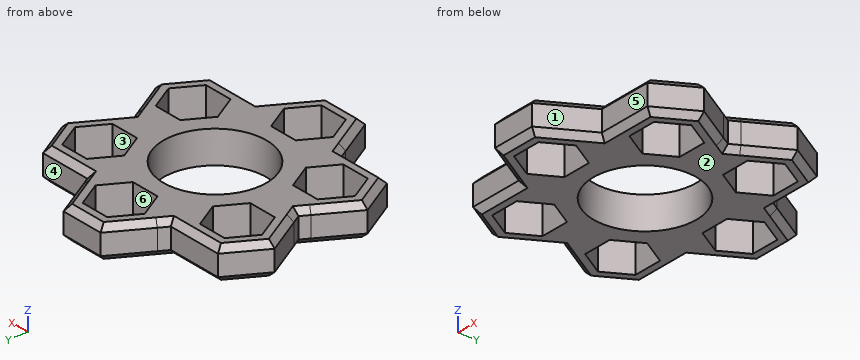
from build123d import *

# Parameters (mm, degrees)
F1_DEPTH = 6.9977
F2_R     = 11.176
F3_DEPTH = 6.9977
F4_SIZE  = 1.27


# Not quite as in the source:
# - a feature names something its author has since deleted; it is built from what else it names


with BuildPart() as f1:
    # F0 (on Top) → F1 (new body)
    with BuildSketch(Plane.XY):
        Polygon((-1.27, 12.7), (1.27, 12.7), (5.4871048633, 12.7), (6.9125849394, 15.169003917), (7.0907659214, 15.4776224307), (9.8865139145, 20.32), (5.1204874424, 28.575), (-4.411565502, 28.575), (-9.1775919741, 20.32), (-4.7781829229, 12.7), align=None)
        Polygon((6.6602806103, 20.32), (3.5073707902, 14.859), (-2.7984488498, 14.859), (-5.9513586699, 20.32), (-2.7984488498, 25.781), (3.5073707902, 25.781), align=None, mode=Mode.SUBTRACT)
        Polygon((6.9125849394, 15.169003917), (5.4871048633, 12.7), (7.3323484187, 12.7), (8.4322006815, 10.795), (12.8316097327, 18.415), (10.9863661773, 18.415), (9.8865139145, 20.32), (7.0907659214, 15.4776224307), align=None)
        Polygon((-7.3323484187, 12.7), (-4.7781829229, 12.7), (-9.1775919741, 20.32), (-10.3250266623, 18.3325848218), (-12.8789355329, 18.3325848218), (-8.4796547943, 10.7128070657), align=None)
        Polygon((12.8316097327, 18.415), (8.4322006815, 10.795), (11.6335226281, 5.2501477372), (13.5648445746, 1.905), (16.3276362049, 1.905), (18.8676362049, 1.905), (22.3636626771, 1.905), (27.1296891492, 10.16), (22.3636626771, 18.415), align=None)
        Polygon((20.7505460249, 4.699), (14.4447263849, 4.699), (11.2918165648, 10.16), (14.4447263849, 15.621), (20.7505460249, 15.621), (23.903455845, 10.16), align=None, mode=Mode.SUBTRACT)
        Polygon((-9.8614826635, 8.3194109889), (-8.4796547943, 10.7128070657), (-12.8789355329, 18.3325848218), (-22.4109884772, 18.3325848218), (-27.1770149494, 10.0775848218), (-22.4109884772, 1.8225848218), (-13.612427, 1.8225848218), (-11.1783483187, 6.0385327673), align=None)
        Polygon((-14.492052185, 15.5385848218), (-11.339142365, 10.0775848218), (-14.492052185, 4.6165848218), (-20.7978718251, 4.6165848218), (-23.9507816452, 10.0775848218), (-20.7978718251, 15.5385848218), align=None, mode=Mode.SUBTRACT)
        Polygon((16.3276362049, 1.905), (13.5648445746, 1.905), (14.6646968374, 0), (13.5648445746, -1.905), (22.3636626771, -1.905), (21.2638104143, 0), (22.3636626771, 1.905), (18.8676362049, 1.905), align=None)
        Polygon((-14.6646968374, 0), (-13.612427, 1.8225848218), (-22.4109884772, 1.8225848218), (-21.311264527, -0.0821929343), (-22.3636626771, -1.905), (-19.9342235854, -1.905), (-17.3764717744, -1.905), (-13.5648445746, -1.905), align=None)
        Polygon((22.3636626771, -1.905), (13.5648445746, -1.905), (10.3635226281, -7.4498522628), (8.4322006815, -10.795), (9.8135964967, -13.1876477372), (11.0835964967, -15.3873522628), (12.8316097327, -18.415), (22.3636626771, -18.415), (27.1296891492, -10.16), align=None)
        Polygon((14.4447263849, -15.621), (11.2918165648, -10.16), (14.4447263849, -4.699), (20.7505460249, -4.699), (23.903455845, -10.16), (20.7505460249, -15.621), align=None, mode=Mode.SUBTRACT)
        Polygon((-11.6335226281, -5.2501477372), (-13.5648445746, -1.905), (-17.3764717744, -1.905), (-19.9342235854, -1.905), (-22.3636626771, -1.905), (-27.1296891492, -10.16), (-22.3636626771, -18.415), (-12.8316097327, -18.415), (-8.4322006815, -10.795), (-10.3635226281, -7.4498522628), align=None)
        Polygon((-20.7505460249, -4.699), (-14.4447263849, -4.699), (-11.2918165648, -10.16), (-14.4447263849, -15.621), (-20.7505460249, -15.621), (-23.903455845, -10.16), align=None, mode=Mode.SUBTRACT)
        Polygon((9.8135964967, -13.1876477372), (8.4322006815, -10.795), (7.3323484187, -12.7), (5.1326438931, -12.7), (9.5320529443, -20.32), (4.7660264722, -28.575), (10.6457036946, -18.415), (12.8316097327, -18.415), (11.0835964967, -15.3873522628), align=None)
        Polygon((9.5320529443, -20.32), (5.1326438931, -12.7), (1.27, -12.7), (-1.27, -12.7), (-5.1326438931, -12.7), (-6.5140397082, -15.0926477372), (-7.7840397082, -17.2923522628), (-9.5320529443, -20.32), (-4.7660264722, -28.575), (4.7660264722, -28.575), align=None)
        Polygon((-6.3058196401, -20.32), (-3.15290982, -14.859), (3.15290982, -14.859), (6.3058196401, -20.32), (3.15290982, -25.781), (-3.15290982, -25.781), align=None, mode=Mode.SUBTRACT)
        Polygon((-7.3323484187, -12.7), (-8.4322006815, -10.795), (-12.8316097327, -18.415), (-10.6319052071, -18.415), (-9.5320529443, -20.32), (-7.7840397082, -17.2923522628), (-6.5140397082, -15.0926477372), (-5.1326438931, -12.7), align=None)
        Polygon((5.4871048633, 12.7), (1.27, 12.7), (-1.27, 12.7), (-4.7781829229, 12.7), (-4.411565502, 12.065), (-2.0086818804, 12.065), (1.267424375, 12.065), (5.1204874424, 12.065), align=None)
        Polygon((-12.8316097327, -1.905), (-13.5648445746, -1.905), (-11.6335226281, -5.2501477372), (-11.0835964967, -4.9326477372), align=None)
        Polygon((1.27, -12.7), (5.1326438931, -12.7), (4.7660264722, -12.065), (1.27, -12.065), (-1.27, -12.065), (-4.7660264722, -12.065), (-5.1326438931, -12.7), (-1.27, -12.7), align=None)
        Polygon((9.8135964967, -7.1323522628), (10.3635226281, -7.4498522628), (11.5783918417, -5.2183179628), (11.0835964967, -4.9326477372), align=None)
        Polygon((11.0835964967, 4.9326477372), (11.6335226281, 5.2501477372), (10.3083918417, 7.4180224884), (9.8135964967, 7.1323522628), align=None)
        Polygon((-9.3113640632, 8.0017998669), (-9.8614826635, 8.3194109889), (-11.1783483187, 6.0385327673), (-10.6282297184, 5.7209216453), align=None)
        Polygon((11.6335226281, 5.2501477372), (8.4322006815, 10.795), (8.0655832606, 10.16), (9.8135964967, 7.1323522628), (10.3083918417, 7.4180224884), align=None)
        Polygon((10.3635226281, -7.4498522628), (13.5648445746, -1.905), (12.8316097327, -1.905), (11.0835964967, -4.9326477372), (11.5783918417, -5.2183179628), align=None)
    extrude(amount=F1_DEPTH)

    # F2 (on Top) → F3 (join)
    with BuildSketch(Plane.XY):
        Polygon((7.6989658396, 13.335), (-7.6989658396, 13.335), (-15.3979316793, 0), (-7.6989658396, -13.335), (7.6989658396, -13.335), (15.3979316793, 0), align=None)
        Circle(F2_R, mode=Mode.SUBTRACT)
    extrude(amount=F3_DEPTH)

    # F4
    f4_edges = [f1.edges().sort_by_distance(p)[0] for p in [
        (-16.497784, -18.415, 6.9977),
        (-16.497784, -18.415, 0),
        (-7.698966, -23.495, 6.9977),
        (-7.698966, -23.495, 0),
        (0, -28.575, 6.9977),
        (0, -28.575, 0),
        (7.705865, -23.495, 0),
        (7.705865, -23.495, 6.9977),
        (16.504683, -18.415, 0),
        (16.504683, -18.415, 6.9977),
        (24.746676, -14.2875, 6.9977),
        (24.746676, -14.2875, 0),
        (24.19675, 5.08, 0),
        (24.19675, 5.08, 6.9977),
        (24.746676, 14.2875, 6.9977),
        (24.746676, 14.2875, 0),
        (16.675014, 18.415, 0),
        (16.675014, 18.415, 6.9977),
        (8.053427, 23.495, 0),
        (8.053427, 23.495, 6.9977),
        (0.354461, 28.575, 0),
        (0.354461, 28.575, 6.9977),
        (-7.368296, 23.453792, 6.9977),
        (-7.368296, 23.453792, 0),
        (-16.368008, 18.332585, 0),
        (-16.368008, 18.332585, 6.9977),
        (-24.794002, 14.205085, 0),
        (-24.794002, 14.205085, 6.9977),
        (-24.24414, 4.997696, 6.9977),
        (-24.24414, 4.997696, 0),
        (-24.220477, -5.121096, 0),
        (-24.220477, -5.121096, 6.9977),
        (-24.746676, -14.2875, 6.9977),
        (-24.746676, -14.2875, 0),
        (24.19675, -5.08, 0),
        (24.19675, -5.08, 6.9977),
    ]]
    chamfer(f4_edges, length=F4_SIZE)


solid = f1.part
Read the model definition and answer for the solid it produces. Units are mm, in the model's axes. Face numbers are marked on the shaded views. A direction names the side the tool comes from. Give positions to 0.01 mm unless a question says otherwise; leave off trailing zeros. Write each loop counter-clockwise with the first axis right and the second up, starting at its lowest first coordinate (ties: lowest second). Pieces come first, ordered by that corner, then holes. Notation, with made-up numbers: (33.25, -11.5) - (46.25, -11.5) arc R22 cw to (46.25, 23.5) - close; hole circle Ø2 at (39, -23). An arc over 180 degrees is marked (long way). Answer in a Markdown table with one row per item. Add a question column.
Item 1: Section B-B, the plane x = 0 is taken. Write down the section's boundary in (y, z) (3 decimals).
Item 2: Find the intervals of material crossed by L1, parallel to Y at x = 0, z = 3 (3 decimals); L2, parallel to X at y = 9.5, z = 2.5; L3, parallel to Y at x = -5.5, z = 5.5, in increasing order.
Item 3: A tool of negligible diameter and unlimited length cuts with its end or side. For the marked faces 4, 5 and 6, from which of +Z, -Z, +X, -X, +Y, -Y can it reach the whole face along a straight path? Write none if from no direction.
Item 4: Section A-A, the plane x = -18.5 is taken. Write down the section's boundary in (y, z) (3 decimals), and give its area (3 significant figures).
Item 5: Section C-C, the plane y = -1 is taken. Write down the section's boundary in (x, z).
Item 6: Flat-ended cylindrical pins translate along their axes: P1, Ø1.9, axis at x = -16.5, z = 5, coming from the +Y side; P2, Ø3, axis at x = 19, z = 5, coming from the -Y side (3 decimals); P3, Ø1.5, axis at y = 17, z = 6, coming from the +X side; P4, Ø12, axis at x = 2, y = 5, coming from the -Z side. Find the tip coordinate at first contact, or state that the pin passes through.
Item 7: Section D-D, the plane y = -13.5 is taken. Write down the section's boundary in (x, z).
Item 8: Determine the mould class of the marked faces 1, 2 and 3 for opening direction Y: pulls with the +Y half, pulls with the -Y half, needs draft (parallel to the pull), parting line crosses it, or undercut.
Recorded:
| question | item | result |
|---|---|---|
| 1 | outline | (-28.575, 1.27) - (-27.305, 0) - (-25.781, 0) - (-25.781, 6.998) - (-27.305, 6.998) - (-28.575, 5.728) - close; (-14.859, 0) - (-11.176, 0) - (-11.176, 6.998) - (-14.859, 6.998) - close; (11.176, 0) - (14.859, 0) - (14.859, 6.998) - (11.176, 6.998) - close; (25.781, 0) - (27.305, 0) - (28.575, 1.27) - (28.575, 5.728) - (27.305, 6.998) - (25.781, 6.998) - close |
| 2 | L1 | y = -28.575 to -25.781, -14.859 to -11.176, 11.176 to 14.859, 25.781 to 28.575 |
| 2 | L2 | x = -26.84 to -23.62, -11.67 to -5.89, 5.89 to 11.67, 23.52 to 26.75 |
| 2 | L3 | y = -27.3 to -21.72, -18.92 to -9.73, 9.73 to 19.54, 21.1 to 26.69 |
| 3 | face 4 | +Z, -Z, +X, +Y |
| 3 | face 5 | +Z, -Z, +X, -Y |
| 3 | face 6 | +Z, -Z |
| 4 | outline | (-18.415, 1.27) - (-17.145, 0) - (-15.621, 0) - (-15.621, 6.998) - (-17.145, 6.998) - (-18.415, 5.728) - close; (-4.699, 0) - (4.617, 0) - (4.617, 6.998) - (-4.699, 6.998) - close; (15.539, 0) - (17.063, 0) - (18.333, 1.27) - (18.333, 5.728) - (17.063, 6.998) - (15.539, 6.998) - close |
| 4 | area | 101 mm2 |
| 5 | outline | (-21.84, 1.27) - (-20.37, 0) - (-11.13, 0) - (-11.13, 7) - (-20.37, 7) - (-21.84, 5.73) - close; (11.13, 0) - (20.37, 0) - (21.84, 1.27) - (21.84, 5.73) - (20.37, 7) - (11.13, 7) - close |
| 6 | P1 | stops at y = 18.33 |
| 6 | P2 | stops at y = -18.415 |
| 6 | P3 | stops at x = 23.58 |
| 6 | P4 | stops at z = 0 |
| 7 | outline | (-25.2, 1.27) - (-23.73, 0) - (-21.98, 0) - (-21.98, 7) - (-23.73, 7) - (-25.2, 5.73) - close; (-13.22, 0) - (13.22, 0) - (13.22, 7) - (-13.22, 7) - close; (21.98, 0) - (23.73, 0) - (25.2, 1.27) - (25.2, 5.73) - (23.73, 7) - (21.98, 7) - close |
| 8 | face 1 | pulls with the -Y half |
| 8 | face 2 | needs draft |
| 8 | face 3 | undercut |
